Design review of the part built by this model. Coordinates are the model's own, in mm. Face numbers are marked on the shaded views. A direction names the side the tool comes from. Give positions to 0.01 mm unless a question says otherwise; leave off trailing zeros. Loops run counter-clockwise (first coordinate to the right, second up) from the corner with the lowest first, then second, coordinate; pieces in that order, holes last. Notation, with made-up numbers: (32.5, 33) -> (51.5, 33) arc R12 cw to (51.5, 38) -> close; hole circle Ø3 at (6.25, -1). An arc over 180 degrees is marked (long way). Use CSV: the item, a comma, the result in double quotes. Start each with the question number.
Item 1: For the marked faces 1, 2 and 3, list the 3-axis set-ups (+Z, -Z, +X, -X, +Y, -Y) from which the entire face can be reached by the end or side of a thin tool; tool diameter is ignored.
Item 2: We need section D-D (y = -2.5). State the section outline as (x, z) points.
Item 3: Clearance check with flat-ended pins moving along their axes: pin 1 (1 mm diameter, centred on x = 0, z = 37, fed in from -Y); pin 2 (4 mm diameter, centred on y = 3.5, z = 25, fed in from +X); pin 3 (2 mm diameter, centred on x = 4, z = 13.5, fed in from -Y). State where each tip first meets the part, or that it passes through.
Item 4: We need section A-A (y = 2.5). State the section outline as (x, z) points, plus the area to 3 significant figures.
Item 5: We need section B-B (z = 17). State the section outline as (x, y) points.
Item 6: Wall thickness on line 1 along Z through (x, y) = (-5.75, -2); line 2 along Y through (x, z) = (0.25, 25.5); line 3 along X through (y, z) = (0, 48): over which ranges is each line inside the solid? List them lowest first. Write a range as from..to.
Item 7: We need section C-C (x = 3). State the section outline as (y, z) points, plus the area to 3 significant figures.
from build123d import *

# Parameters (mm, degrees)
SKETCH_1_R      = 4
EXTRUDE_1_DEPTH = 50
EXTRUDE_START   = -8
SKETCH_2_R      = 7
EXTRUDE_2_DEPTH = 4


with BuildPart() as part:
    # 草图1 → 凸台-拉伸1 (new body)
    with BuildSketch(Plane.XY):
        Circle(SKETCH_1_R)
    extrude(amount=EXTRUDE_1_DEPTH)

    # 草图2 → 凸台-拉伸2 (add)
    with BuildSketch(Plane.XY.offset(50).offset(EXTRUDE_START)):
        Circle(SKETCH_2_R)
    extrude(amount=-EXTRUDE_2_DEPTH)

    # 草图4 → 切除-旋转1 (revolve, cut)
    with BuildSketch(Plane(origin=(0, 0, 0), x_dir=(0, 0, -1), z_dir=(1, 0, 0)), mode=Mode.PRIVATE) as cut_revolve_1_sk:
        Polygon((-2.6, -4.84176312), (-4, -4.84176312), (-4, 4.751502862), (-2.5, 4.751502862), align=None)
    revolve(cut_revolve_1_sk.sketch.rotate(Axis((0, 6.786956164, 4), (0, -1, 0)), 311.656275419), axis=Axis((0, 6.786956164, 4), (0, -1, 0)), mode=Mode.SUBTRACT)


solid = part.part
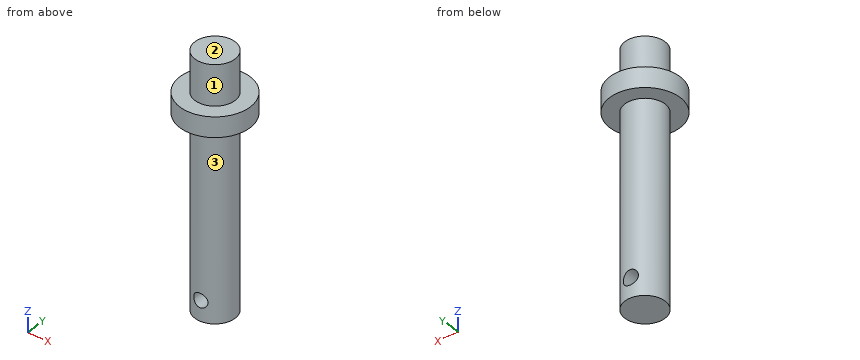
Results found:
1,face 1,"+Z"
1,face 2,"+Z, +X, -X, +Y, -Y"
1,face 3,"-Z"
2,outline,"(-6.54, 38) -> (-3.12, 38) -> (-3.12, 0) -> (3.12, 0) -> (3.12, 38) -> (6.54, 38) -> (6.54, 42) -> (3.12, 42) -> (3.12, 50) -> (-3.12, 50) -> (-3.12, 42) -> (-6.54, 42) -> close; hole circle Ø2.85 at (0, 4)"
3,pin 1,"y = -4"
3,pin 2,"x = 3.71"
3,pin 3,"y = -2.65"
4,outline,"(-6.54, 38) -> (-3.12, 38) -> (-3.12, 0) -> (3.12, 0) -> (3.12, 38) -> (6.54, 38) -> (6.54, 42) -> (3.12, 42) -> (3.12, 50) -> (-3.12, 50) -> (-3.12, 42) -> (-6.54, 42) -> close; hole circle Ø2.95 at (0, 4)"
4,area,"333 mm²"
5,outline,"circle Ø8 at (0, 0)"
6,line 1,"38..42"
6,line 2,"-3.99..3.99"
6,line 3,"-4..4"
7,outline,"(-6.32, 38) -> (-2.65, 38) -> (-2.65, 0) -> (2.65, 0) -> (2.65, 38) -> (6.32, 38) -> (6.32, 42) -> (2.65, 42) -> (2.65, 50) -> (-2.65, 50) -> (-2.65, 42) -> (-6.32, 42) -> close"
7,area,"294 mm²"
